from build123d import *

# Parameters (mm, degrees)
SKETCH1_W                      = 424.942
SKETCH1_H                      = 121.412
SKETCH1_R                      = 1.8288
BASE_FLANGE1_DEPTH             = 2.286
SKETCH4_W                      = 0.0254
SKETCH4_H                      = 0.254
SKETCH4_W_2                    = 0.254
CUT_EXTRUDE1_DEPTH             = 2.286
EDGE_FLANGE1_STRIP_W           = 9.4488
EDGE_FLANGE1_STRIP_H           = 2.286
EDGE_FLANGE1_STRIP_CUT_DEPTH   = 390.1186
EDGE_FLANGE1_STRIP_2_W         = 9.4488
EDGE_FLANGE1_STRIP_2_H         = 2.286
EDGE_FLANGE1_STRIP_CUT_2_DEPTH = 390.1186
EDGE_FLANGE1_DEPTH             = 390.1186
EDGE_FLANGE1_BEND_DEPTH        = 390.1186
SKETCH10_R                     = 2.3876
CUT_EXTRUDE2_DEPTH             = 443.175190715


# Sheet-metal steps are written as plain solids
with BuildPart() as part:
    # Sketch1 → Base-Flange1 (new body)
    with BuildSketch(Plane.XY):
        with Locations((212.471, 60.706)):
            Rectangle(SKETCH1_W, SKETCH1_H)
        with Locations((9.906, 13.081)):
            Circle(SKETCH1_R, mode=Mode.SUBTRACT)
        with Locations((415.036, 13.081)):
            Circle(SKETCH1_R, mode=Mode.SUBTRACT)
        with Locations((9.906, 108.331)):
            Circle(SKETCH1_R, mode=Mode.SUBTRACT)
        with Locations((415.036, 108.331)):
            Circle(SKETCH1_R, mode=Mode.SUBTRACT)
    extrude(amount=-BASE_FLANGE1_DEPTH)

    # Sketch4 → Cut-Extrude1 (cut)
    with BuildSketch(Plane.XY):
        with Locations((17.2847, 121.285)):
            Rectangle(SKETCH4_W, SKETCH4_H)
        with Locations((407.543, 121.285)):
            Rectangle(SKETCH4_W_2, SKETCH4_H)
        with Locations((407.543, 0.127)):
            Rectangle(SKETCH4_W_2, SKETCH4_H)
        with Locations((17.2847, 0.127)):
            Rectangle(SKETCH4_W, SKETCH4_H)
    extrude(amount=-CUT_EXTRUDE1_DEPTH, mode=Mode.SUBTRACT)

    # Edge-Flange1 strip (across the edge) → Edge-Flange1 strip cut (cut)
    with BuildSketch(Plane(origin=(407.416, 121.412, 0), x_dir=(0, -1, 0), z_dir=(-1, 0, 0))):
        with Locations((-2.286, -1.143)):
            Rectangle(EDGE_FLANGE1_STRIP_W, EDGE_FLANGE1_STRIP_H)
    extrude(amount=EDGE_FLANGE1_STRIP_CUT_DEPTH, mode=Mode.SUBTRACT)

    # Edge-Flange1 strip 2 (across the edge) → Edge-Flange1 strip cut 2 (cut)
    with BuildSketch(Plane.YZ.offset(17.2974)):
        with Locations((-2.286, -1.143)):
            Rectangle(EDGE_FLANGE1_STRIP_2_W, EDGE_FLANGE1_STRIP_2_H)
    extrude(amount=EDGE_FLANGE1_STRIP_CUT_2_DEPTH, mode=Mode.SUBTRACT)

    # Edge-Flange1 section (across the edge) → Edge-Flange1 (add)
    with BuildSketch(Plane(origin=(407.416, 121.412, 0), x_dir=(0, -1, 0), z_dir=(-1, 0, 0))):
        with BuildLine():
            Line((0, 0.1524), (0, 14.224))
            Line((0, 14.224), (2.286, 14.224))
            Line((2.286, 14.224), (2.286, 0.1524))
            ThreePointArc((2.286, 0.1524), (2.330636927, 0.044636927), (2.4384, 0))
            Line((2.4384, 0), (2.4384, -2.286))
            ThreePointArc((2.4384, -2.286), (0.714190825, -1.571809175), (0, 0.1524))
        make_face()
    extrude(amount=EDGE_FLANGE1_DEPTH)

    # Edge-Flange1 section 2 (across the edge) → Edge-Flange1 bend (add)
    with BuildSketch(Plane.YZ.offset(17.2974)):
        with BuildLine():
            Line((0, 0.1524), (0, 14.224))
            Line((0, 14.224), (2.286, 14.224))
            Line((2.286, 14.224), (2.286, 0.1524))
            ThreePointArc((2.286, 0.1524), (2.330636927, 0.044636927), (2.4384, 0))
            Line((2.4384, 0), (2.4384, -2.286))
            ThreePointArc((2.4384, -2.286), (0.714190825, -1.571809175), (0, 0.1524))
        make_face()
    extrude(amount=EDGE_FLANGE1_BEND_DEPTH)

    # Sketch10 → Cut-Extrude2 (cut, through all)
    with BuildSketch(Plane(origin=(0, 121.412, 0), x_dir=(-1, 0, 0), z_dir=(0, 1, 0))):
        with Locations(Location((-402.971, 7.112, 0), (0, 0, 90))):
            Circle(SKETCH10_R)
        with Locations(Location((-275.971, 7.112, 0), (0, 0, 90))):
            Circle(SKETCH10_R)
        with Locations(Location((-148.971, 7.112, 0), (0, 0, 90))):
            Circle(SKETCH10_R)
        with Locations(Location((-21.971, 7.112, 0), (0, 0, 90))):
            Circle(SKETCH10_R)
    extrude(amount=-CUT_EXTRUDE2_DEPTH, mode=Mode.SUBTRACT)


solid = part.part
The model under review builds one solid part; all positions refer to its coordinate system, in mm. A direction names the side the tool comes from. Round coordinates to 2 decimals unless told otherwise and drop trailing zeros. Write each loop counter-clockwise with the first axis right and the second up, starting at its lowest first coordinate (ties: lowest second). Pieces come first, ordered by that corner, then holes. Notation, with made-up numbers: M -28.75,46 L -18.75,46 A15 ccw -18.75,53 Z; hole C 40,-11.5 d8. An arc over 180 degrees is marked long. Answer as CSV lines item,"result". Start each with the question number.
Q1. The part is to be moulded in two halves that separate along Y. For faces 3 (the face through (215, 119.126, 7)), 4 (the face through (210, 0, 7)), 5 (the face through (215, 121.412, 7)), 6 (the face through (209, 62, 0)), say which applies: +Y half, -Y half, draft (parallel to the pull), parting line (faces both ways), or undercut.
Q2. Wall thickness on line 1 along Y through (x, z) = (265, 5.25); line 2 along Z through (x, y) = (381, 110): over which ranges is each line inside the solid? List them lowest first.
Q3. Clearance check with flat-ended pins moving along their axes: P1, Ø2, axis at y = 1, z = 6, coming from the +X side; P2, Ø10, axis at x = 224.5, y = 49, coming from the +Z side. State where each tip first meets the part, or that it passes through.
Q4. Consider section A-A, the plane x = 67.5. Give the boundary of the cut face in (y, z), then the cut area to 3 significant figures.
Q5. Tool access review of faces 1 (the face through (209, 62, -2.286)), 2 (the face through (210, 2.286, 7)): name each direction out of +Z, -Z, +X, -X, +Y, -Y from which nothing blocks a thin tool from reaching the whole face with its end or side.
Q6. Consider section B-B, the plane y = 80. Give the boundary of the cut face in (x, z).
Result set:
1,face 3,"undercut"
1,face 4,"-Y half"
1,face 5,"+Y half"
1,face 6,"undercut"
2,line 1,"y = 0 to 2.29, 119.13 to 121.41"
2,line 2,"z = -2.29 to 0"
3,P1,"stops at x = 407.42"
3,P2,"stops at z = 0"
4,outline,"M 0,0.15 A2.44 ccw 2.44,-2.29 L 118.97,-2.29 A2.44 ccw 121.41,0.15 L 121.41,14.22 L 119.13,14.22 L 119.13,0.15 A0.15 cw 118.97,0 L 2.44,0 A0.15 cw 2.29,0.15 L 2.29,14.22 L 0,14.22 Z"
4,area,"340 mm²"
5,face 1,"-Z, +X, -X, +Y, -Y"
5,face 2,"+Z, +X, -X"
6,outline,"M 0,-2.29 L 424.94,-2.29 L 424.94,0 L 0,0 Z"
